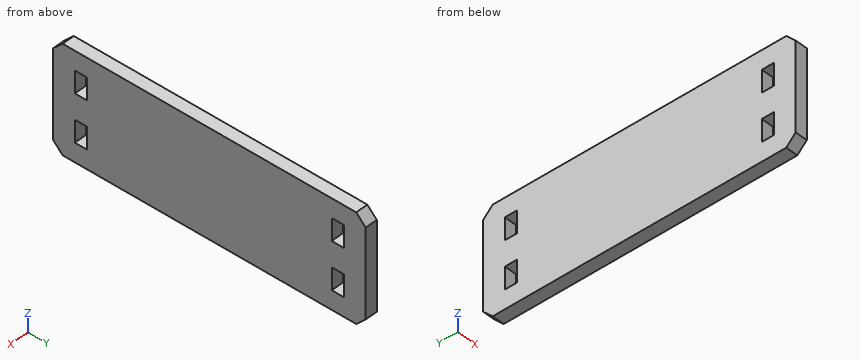
from build123d import *

# Parameters (mm, degrees)
SKETCH1_W           = 43.18
SKETCH1_H           = 126.492
SKETCH1_W_2         = 8.89
SKETCH1_H_2         = 4.953
BOSS_EXTRUDE1_DEPTH = 2.4765
CHAMFER1_SIZE       = 3.81


with BuildPart() as part:
    # Sketch1 → Boss-Extrude1 (new body, symmetric)
    with BuildSketch(Plane(origin=(0, 0, 0), x_dir=(0, 0, -1), z_dir=(1, 0, 0))):
        with Locations((-111.027292876, 0)):
            Rectangle(SKETCH1_W, SKETCH1_H)
        with Locations((-101.502292876, 52.0065)):
            Rectangle(SKETCH1_W_2, SKETCH1_H_2, mode=Mode.SUBTRACT)
        with Locations((-120.552292876, 52.0065)):
            Rectangle(SKETCH1_W_2, SKETCH1_H_2, mode=Mode.SUBTRACT)
        with Locations((-101.502292876, -52.0065)):
            Rectangle(SKETCH1_W_2, SKETCH1_H_2, mode=Mode.SUBTRACT)
        with Locations((-120.552292876, -52.0065)):
            Rectangle(SKETCH1_W_2, SKETCH1_H_2, mode=Mode.SUBTRACT)
    extrude(amount=BOSS_EXTRUDE1_DEPTH, both=True)

    # Chamfer1
    chamfer1_edges = [part.edges().sort_by_distance(p)[0] for p in [
        (0, -63.246, 89.437292876),
        (0, -63.246, 132.617292876),
        (0, 63.246, 132.617292876),
        (0, 63.246, 89.437292876),
    ]]
    chamfer(chamfer1_edges, length=CHAMFER1_SIZE)


solid = part.part
Source: CAD feature listing. Evaluate the final solid. Frame: model axes, mm. Coordinates: 2 decimals unless noted, no trailing zeros. Loops run counter-clockwise (first coordinate to the right, second up) from the corner with the lowest first, then second, coordinate; pieces in that order, holes last. Notation, with made-up numbers: M 55.5,18 L 81.5,18 A26 cw 81.5,56 Z; hole C 31,19 d4. An arc over 180 degrees is marked long. Answer in a Markdown table with one row per item.
Q1. Section B-B on x = 1.6. Return the cut outline in (y, z).
Answers below:
| item | result |
|---|---|
| outline | M -63.25,93.25 L -59.44,89.44 L 59.44,89.44 L 63.25,93.25 L 63.25,128.81 L 59.44,132.62 L -59.44,132.62 L -63.25,128.81 Z; hole M -54.48,97.06 L -49.53,97.06 L -49.53,105.95 L -54.48,105.95 Z; hole M -54.48,116.11 L -49.53,116.11 L -49.53,125 L -54.48,125 Z; hole M 49.53,97.06 L 54.48,97.06 L 54.48,105.95 L 49.53,105.95 Z; hole M 49.53,116.11 L 54.48,116.11 L 54.48,125 L 49.53,125 Z |
Q2. Section A-A on z = 118.5. Return the cut outline in (x, y), plus the area to 3 significant figures.
Answers below:
| item | result |
|---|---|
| outline | M -2.48,-63.25 L 2.48,-63.25 L 2.48,-54.48 L -2.48,-54.48 Z; M -2.48,-49.53 L 2.48,-49.53 L 2.48,49.53 L -2.48,49.53 Z; M -2.48,54.48 L 2.48,54.48 L 2.48,63.25 L -2.48,63.25 Z |
| area | 577 mm^2 |
Q3. Ray query, probe 1 along Y at (x, z) = (-0.6, 117); probe 2 along Z at (x, y) = (0.15, 50). Return the intervals inside material, ascending. Write a range as from..to.
Answers below:
| item | result |
|---|---|
| probe 1 | y = -63.25..-54.48, -49.53..49.53, 54.48..63.25 |
| probe 2 | z = 89.44..97.06, 105.95..116.11, 125..132.62 |
